Input: part model. Units: mm. Frame: model coordinates. Coordinates: 2 decimals unless noted, no trailing zeros. Loops run counter-clockwise (first coordinate to the right, second up) from the corner with the lowest first, then second, coordinate; pieces in that order, holes last. Notation, with made-up numbers: (58, 39.5) - (71, 39.5) arc R24 cw to (71, 60.5) - close; hole circle Ø11 at (78, -0.75). An arc over 180 degrees is marked (long way). Use a Markdown table: item, result. Add a question column.
1. Section query B-B on y = 15. Return the cut outline in (x, z) (3 decimals), then the cut area to 3 significant figures.
2. Ray query, L1, parallel to X at y = 50, z = -1; L2, parallel to X at y = 67.5, z = -3.05; L3, parallel to Z at x = -46, y = 33.5 (3 decimals). Return the intervals inside material, ascending. Write a range as [from, to].
3. Section query A-A on y = -2.5. Return the cut outline in (x, z) (3 decimals).
4. Contact query for a flat-ended pin moving along its axis: P1, Ø8.5, axis at x = 50, y = 67.5, coming from the +Z side. Output: stop coordinate, or through.
```python
from build123d import *

# Parameters (mm, degrees)
BASE_FLANGE1_START                           = -4.375
BASE_FLANGE1_OUTLINE_W                       = 130
BASE_FLANGE1_OUTLINE_H                       = 170
BASE_FLANGE1_DEPTH                           = 8.75
M6_TAPPED_HOLE1_AT_2_COUNT                   = 2
M6_TAPPED_HOLE1_AT_2_PITCH                   = 105
M6_TAPPED_HOLE1_AT_3_COUNT                   = 2
M6_TAPPED_HOLE1_AT_3_PITCH                   = 70
M6_TAPPED_HOLE1_AT_4_COUNT                   = 2
M6_TAPPED_HOLE1_AT_4_PITCH                   = 35
CSK_FOR_M6_HEX_SOCKET_COUNTERSUNK_HE_2_COUNT = 2
CSK_FOR_M6_HEX_SOCKET_COUNTERSUNK_HE_2_PITCH = 35
CSK_FOR_M6_HEX_SOCKET_COUNTERSUNK_HE_3_COUNT = 2
CSK_FOR_M6_HEX_SOCKET_COUNTERSUNK_HE_3_PITCH = 70
CSK_FOR_M6_HEX_SOCKET_COUNTERSUNK_HE_4_COUNT = 2
CSK_FOR_M6_HEX_SOCKET_COUNTERSUNK_HE_4_PITCH = 105
CSK_FOR_M6_HEX_SOCKET_COUNTERSUNK_HE_5_COUNT = 2
CSK_FOR_M6_HEX_SOCKET_COUNTERSUNK_HE_5_PITCH = 140
FILLET1_R                                    = 2
CHAMFER1_SIZE                                = 0.8


# Read off the part's stored shape, not the designer's step: Base-Flange1
with BuildPart() as part:
    # Base-Flange1 outline → Base-Flange1 (new body)
    with BuildSketch(Plane.XY.offset(BASE_FLANGE1_START)):
        Rectangle(BASE_FLANGE1_OUTLINE_W, BASE_FLANGE1_OUTLINE_H)
    extrude(amount=BASE_FLANGE1_DEPTH)

    # Sketch8 → M6 Tapped Hole1 (revolve, cut)
    with BuildSketch(Plane(origin=(-47.5, -55, 4.375), x_dir=(0, -1, 0), z_dir=(1, 0, 0))):
        Polygon((0, 0), (0, 8.75), (3, 8.75), (2.5, 8.25), (2.5, 0.5), (3, 0), align=None)
    m6_tapped_hole1 = revolve(axis=Axis((-47.5, -55, 10.725), (0, 0, -1)), mode=Mode.SUBTRACT)

    # M6 Tapped Hole1 at 2: M6 Tapped Hole1 ×2
    with Locations(*[(0, i * M6_TAPPED_HOLE1_AT_2_PITCH, 0) for i in range(1, M6_TAPPED_HOLE1_AT_2_COUNT)]):
        add(m6_tapped_hole1, mode=Mode.SUBTRACT)

    # M6 Tapped Hole1 at 3: M6 Tapped Hole1 ×2
    with Locations(*[(0, i * M6_TAPPED_HOLE1_AT_3_PITCH, 0) for i in range(1, M6_TAPPED_HOLE1_AT_3_COUNT)]):
        add(m6_tapped_hole1, mode=Mode.SUBTRACT)

    # M6 Tapped Hole1 at 4: M6 Tapped Hole1 ×2
    with Locations(*[(0, i * M6_TAPPED_HOLE1_AT_4_PITCH, 0) for i in range(1, M6_TAPPED_HOLE1_AT_4_COUNT)]):
        add(m6_tapped_hole1, mode=Mode.SUBTRACT)

    # Sketch12 → CSK for M6 Hex Socket Countersunk Head Screw1 (revolve, cut)
    with BuildSketch(Plane(origin=(-50, -72.5, 4.375), x_dir=(0, -1, 0), z_dir=(1, 0, 0))):
        Polygon((0, 0), (0, 8.75), (3.5, 8.75), (3.3, 8.55), (3.3, 3.555), (6.855, 0), align=None)
    csk_for_m6_hex_socket_countersunk_head_s = revolve(axis=Axis((-50, -72.5, 10.725), (0, 0, -1)), mode=Mode.SUBTRACT)

    # CSK for M6 Hex Socket Countersunk He 2: CSK for M6 Hex Socket Countersunk Head Screw1 ×2
    with Locations(*[(0, i * CSK_FOR_M6_HEX_SOCKET_COUNTERSUNK_HE_2_PITCH, 0) for i in range(1, CSK_FOR_M6_HEX_SOCKET_COUNTERSUNK_HE_2_COUNT)]):
        add(csk_for_m6_hex_socket_countersunk_head_s, mode=Mode.SUBTRACT)

    # CSK for M6 Hex Socket Countersunk He 3: CSK for M6 Hex Socket Countersunk Head Screw1 ×2
    with Locations(*[(0, i * CSK_FOR_M6_HEX_SOCKET_COUNTERSUNK_HE_3_PITCH, 0) for i in range(1, CSK_FOR_M6_HEX_SOCKET_COUNTERSUNK_HE_3_COUNT)]):
        add(csk_for_m6_hex_socket_countersunk_head_s, mode=Mode.SUBTRACT)

    # CSK for M6 Hex Socket Countersunk He 4: CSK for M6 Hex Socket Countersunk Head Screw1 ×2
    with Locations(*[(0, i * CSK_FOR_M6_HEX_SOCKET_COUNTERSUNK_HE_4_PITCH, 0) for i in range(1, CSK_FOR_M6_HEX_SOCKET_COUNTERSUNK_HE_4_COUNT)]):
        add(csk_for_m6_hex_socket_countersunk_head_s, mode=Mode.SUBTRACT)

    # CSK for M6 Hex Socket Countersunk He 5: CSK for M6 Hex Socket Countersunk Head Screw1 ×2
    with Locations(*[(0, i * CSK_FOR_M6_HEX_SOCKET_COUNTERSUNK_HE_5_PITCH, 0) for i in range(1, CSK_FOR_M6_HEX_SOCKET_COUNTERSUNK_HE_5_COUNT)]):
        add(csk_for_m6_hex_socket_countersunk_head_s, mode=Mode.SUBTRACT)

    # Mirror1: M6 Tapped Hole1, CSK for M6 Hex Socket Countersunk Head Screw1 across plane
    add(m6_tapped_hole1.mirror(Plane(origin=(0, 0, 0), x_dir=(0, 0, 1), z_dir=(1, 0, 0))), mode=Mode.SUBTRACT)
    add(csk_for_m6_hex_socket_countersunk_head_s.mirror(Plane(origin=(0, 0, 0), x_dir=(0, 0, 1), z_dir=(1, 0, 0))), mode=Mode.SUBTRACT)

    # Mirror1 copy 1 sketch → Mirror1 copy 1 (revolve, cut)
    with BuildSketch(Plane(origin=(47.5, 50, 4.375), x_dir=(0, -1, 0), z_dir=(-1, 0, 0))):
        Polygon((0, 0), (0, -8.75), (3, -8.75), (2.5, -8.25), (2.5, -0.5), (3, 0), align=None)
    revolve(axis=Axis((47.5, 50, 10.725), (0, 0, 1)), mode=Mode.SUBTRACT)

    # Mirror1 copy 2 sketch → Mirror1 copy 2 (revolve, cut)
    with BuildSketch(Plane(origin=(47.5, 15, 4.375), x_dir=(0, -1, 0), z_dir=(-1, 0, 0))):
        Polygon((0, 0), (0, -8.75), (3, -8.75), (2.5, -8.25), (2.5, -0.5), (3, 0), align=None)
    revolve(axis=Axis((47.5, 15, 10.725), (0, 0, 1)), mode=Mode.SUBTRACT)

    # Mirror1 copy 3 sketch → Mirror1 copy 3 (revolve, cut)
    with BuildSketch(Plane(origin=(47.5, -20, 4.375), x_dir=(0, -1, 0), z_dir=(-1, 0, 0))):
        Polygon((0, 0), (0, -8.75), (3, -8.75), (2.5, -8.25), (2.5, -0.5), (3, 0), align=None)
    revolve(axis=Axis((47.5, -20, 10.725), (0, 0, 1)), mode=Mode.SUBTRACT)

    # Mirror1 copy 4 sketch → Mirror1 copy 4 (revolve, cut)
    with BuildSketch(Plane(origin=(50, -37.5, 4.375), x_dir=(0, -1, 0), z_dir=(-1, 0, 0))):
        Polygon((0, 0), (0, -8.75), (3.5, -8.75), (3.3, -8.55), (3.3, -3.555), (6.855, 0), align=None)
    revolve(axis=Axis((50, -37.5, 10.725), (0, 0, 1)), mode=Mode.SUBTRACT)

    # Mirror1 copy 5 sketch → Mirror1 copy 5 (revolve, cut)
    with BuildSketch(Plane(origin=(50, -2.5, 4.375), x_dir=(0, -1, 0), z_dir=(-1, 0, 0))):
        Polygon((0, 0), (0, -8.75), (3.5, -8.75), (3.3, -8.55), (3.3, -3.555), (6.855, 0), align=None)
    revolve(axis=Axis((50, -2.5, 10.725), (0, 0, 1)), mode=Mode.SUBTRACT)

    # Mirror1 copy 6 sketch → Mirror1 copy 6 (revolve, cut)
    with BuildSketch(Plane(origin=(50, 32.5, 4.375), x_dir=(0, -1, 0), z_dir=(-1, 0, 0))):
        Polygon((0, 0), (0, -8.75), (3.5, -8.75), (3.3, -8.55), (3.3, -3.555), (6.855, 0), align=None)
    revolve(axis=Axis((50, 32.5, 10.725), (0, 0, 1)), mode=Mode.SUBTRACT)

    # Mirror1 copy 7 sketch → Mirror1 copy 7 (revolve, cut)
    with BuildSketch(Plane(origin=(50, 67.5, 4.375), x_dir=(0, -1, 0), z_dir=(-1, 0, 0))):
        Polygon((0, 0), (0, -8.75), (3.5, -8.75), (3.3, -8.55), (3.3, -3.555), (6.855, 0), align=None)
    revolve(axis=Axis((50, 67.5, 10.725), (0, 0, 1)), mode=Mode.SUBTRACT)

    # Fillet1
    fillet1_edges = [part.edges().sort_by_distance(p)[0] for p in [
        (-65, 85, 0),
        (65, 85, 0),
        (65, -85, 0),
        (-65, -85, 0),
    ]]
    fillet(fillet1_edges, radius=FILLET1_R)

    # Chamfer1
    chamfer1_edges = [part.edges().sort_by_distance(p)[0] for p in [
        (65, 0, 4.375),
        (65, 0, -4.375),
        (-65, 0, 4.375),
        (0, -85, 4.375),
        (0, 85, 4.375),
        (-64.414213562, 84.414213562, 4.375),
        (-64.414213562, -84.414213562, 4.375),
        (64.414213562, -84.414213562, 4.375),
        (64.414213562, 84.414213562, 4.375),
        (0, 85, -4.375),
        (-65, 0, -4.375),
        (0, -85, -4.375),
        (-64.414213562, 84.414213562, -4.375),
        (-64.414213562, -84.414213562, -4.375),
        (64.414213562, -84.414213562, -4.375),
        (64.414213562, 84.414213562, -4.375),
    ]]
    chamfer(chamfer1_edges, length=CHAMFER1_SIZE)


solid = part.part
```
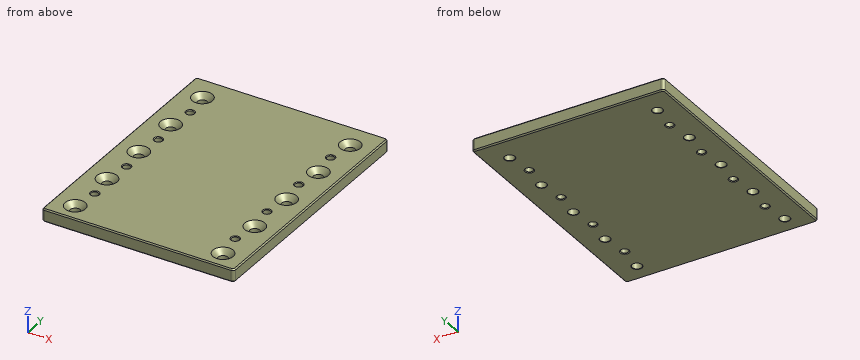
Resolved:
| question | item | result |
|---|---|---|
| 1 | outline | (-65, -3.575) - (-64.2, -4.375) - (-50.5, -4.375) - (-50, -3.875) - (-50, 3.875) - (-50.5, 4.375) - (-64.2, 4.375) - (-65, 3.575) - close; (-45, -3.875) - (-44.5, -4.375) - (44.5, -4.375) - (45, -3.875) - (45, 3.875) - (44.5, 4.375) - (-44.5, 4.375) - (-45, 3.875) - close; (50, -3.875) - (50.5, -4.375) - (64.2, -4.375) - (65, -3.575) - (65, 3.575) - (64.2, 4.375) - (50.5, 4.375) - (50, 3.875) - close |
| 1 | area | 1,050 mm² |
| 2 | L1 | [-65, -50], [-45, 45], [50, 65] |
| 2 | L2 | [-65, -53.3], [-46.7, 46.7], [53.3, 65] |
| 2 | L3 | [-4.375, 1.643] |
| 3 | outline | (-65, -3.575) - (-64.2, -4.375) - (-53.5, -4.375) - (-53.3, -4.175) - (-53.3, 0.82) - (-56.855, 4.375) - (-64.2, 4.375) - (-65, 3.575) - close; (-46.7, -4.175) - (-46.5, -4.375) - (46.5, -4.375) - (46.7, -4.175) - (46.7, 0.82) - (43.145, 4.375) - (-43.145, 4.375) - (-46.7, 0.82) - close; (53.3, -4.175) - (53.5, -4.375) - (64.2, -4.375) - (65, -3.575) - (65, 3.575) - (64.2, 4.375) - (56.855, 4.375) - (53.3, 0.82) - close |
| 4 | P1 | z = 1.77 |
